Could you check a few things on this model? Use its own coordinates, in mm. A direction names the side the tool comes from. Coordinates: 2 decimals unless noted, no trailing zeros. Write each loop counter-clockwise with the first axis right and the second up, starting at its lowest first coordinate (ties: lowest second). Pieces come first, ordered by that corner, then holes.
Item 1: If I drill on probe 1 along X at (y, z) = (17.5, 9.25); probe 2 along X at (y, z) = (20.5, 3.25), over which ranges is the centre line in solid material (lowest first)?
Item 2: Thinking about a two-plate mould opening in Y: for faces 6 (the cylindrical face through (-22.99, 23.02, 8.3)), 7 (the flat face through (-0.2, 23.2, 10.16)), 8 (the cylindrical face through (-20.609, -17.214, 0.376)), which applies, +Y half, -Y half, draft (parallel to the pull), parting line (faces both ways), or undercut?
Item 3: For P1, Ø5, axis at x = -1.5, y = -7.5, coming from the -Z side; P2, Ø1.2, axis at y = -2, z = 0.5, coming from the -X side; P3, Ø1.7, axis at x = 5.5, z = 0.5, coming from the +Y side; P4, Ø0.8, axis at y = -4.5, z = 2, coming from the -X side, each with a flat end and sliding along its axis, tell me the tip position at first contact or that it passes through.
Item 4: Which directions (+Z, -Z, +X, -X, +Y, -Y) give clear straight access to the entire face, cutting with the end or side of a thin tool? Please do faces 1 (the flat face through (-10, 0, 2.54)), 2 (the flat face through (-6.35, -23, 13)), 3 (the flat face through (0, 22.987, 11)), 4 (the cylindrical face through (-14.86, 13.31, 0.38)), 5 (the flat face through (-25, -19.685, 13)).
Item 5: I want a section at C-C on z = 3.75. Please give me the cut outline in (x, y), then the cut area to 3 significant figures.
Item 6: I want a section at D-D on x = 12. Please give me the cut outline in (y, z) (3 decimals).
Item 7: I want a section at A-A on z = 10.75. State how many separate pieces and enclosed holes the cut face has, then the cut area to 3 significant figures.
from build123d import *

# Parameters (mm, degrees)
BOSS_EXTRUDE1_DEPTH             = 14.224
CUT_EXTRUDE1_DEPTH              = 11.684
FILLET1_R                       = 2.54
CUT_EXTRUDE2_DEPTH              = 55.976332917
CUT_EXTRUDE2_DEPTH_BACK         = 55.976332917
SKETCH3_W                       = 32.258
SKETCH3_H                       = 8.128
SKETCH5_W                       = 26.924
SKETCH5_H                       = 34.29
CUT_EXTRUDE4_DEPTH              = 1.524
SKETCH6_W                       = 16.764
SKETCH6_H                       = 24.13
CUT_EXTRUDE5_DEPTH              = 1.524
SKETCH8_W                       = 12.7
SKETCH8_H                       = 0.508
BOSS_EXTRUDE3_DEPTH             = 4.064
SKETCH9_W                       = 12.7
SKETCH9_H                       = 1.016
BOSS_EXTRUDE4_DEPTH             = 0.762
FILLET2_R                       = 0.762
SKETCH10_W                      = 12.7
SKETCH10_H                      = 1.016
BOSS_EXTRUDE5_DEPTH             = 0.762
FILLET3_R                       = 0.762
SKETCH11_W                      = 1.778
SKETCH11_H                      = 4.064
BOSS_EXTRUDE6_DEPTH             = 3.556
BOSS_EXTRUDE6_DIRECTION_2_REACH = 56.976
FILLET4_RADIUS                  = 2.032
FILLET4_LENGTH                  = 1.778
SKETCH12_R                      = 1.143
CUT_EXTRUDE7_DEPTH              = 4.064
CUT_EXTRUDE8_DEPTH              = 0.762


with BuildPart() as part:
    # Sketch1 → Boss-Extrude1 (new body)
    with BuildSketch(Plane.XY):
        with BuildLine():
            Line((-21.209, -23.749), (21.209, -23.749))
            ThreePointArc((21.209, -23.749), (23.005051224, -23.005051224), (23.749, -21.209))
            Line((23.749, -21.209), (23.749, 21.209))
            ThreePointArc((23.749, 21.209), (23.005051224, 23.005051224), (21.209, 23.749))
            Line((21.209, 23.749), (-21.209, 23.749))
            ThreePointArc((-21.209, 23.749), (-23.005051224, 23.005051224), (-23.749, 21.209))
            Line((-23.749, 21.209), (-23.749, -21.209))
            ThreePointArc((-23.749, -21.209), (-23.005051224, -23.005051224), (-21.209, -23.749))
        make_face()
    extrude(amount=BOSS_EXTRUDE1_DEPTH)

    # Sketch2 → Cut-Extrude1 (cut)
    with BuildSketch(Plane.XY.offset(14.224)):
        with BuildLine():
            Line((19.939, -22.479), (-19.939, -22.479))
            ThreePointArc((-19.939, -22.479), (-21.735051224, -21.735051224), (-22.479, -19.939))
            Line((-22.479, -19.939), (-22.479, 19.939))
            ThreePointArc((-22.479, 19.939), (-21.735051224, 21.735051224), (-19.939, 22.479))
            Line((-19.939, 22.479), (19.939, 22.479))
            ThreePointArc((19.939, 22.479), (21.735051224, 21.735051224), (22.479, 19.939))
            Line((22.479, 19.939), (22.479, -19.939))
            ThreePointArc((22.479, -19.939), (21.735051224, -21.735051224), (19.939, -22.479))
        make_face()
    extrude(amount=-CUT_EXTRUDE1_DEPTH, mode=Mode.SUBTRACT)

    # Fillet1
    fillet1_edges = [part.edges().sort_by_distance(p)[0] for p in [
        (0, -23.749, 0),
        (-23.005051224, -23.005051224, 0),
        (-23.749, 0, 0),
        (-23.005051224, 23.005051224, 0),
        (0, 23.749, 0),
        (23.005051224, 23.005051224, 0),
        (23.749, 0, 0),
        (23.005051224, -23.005051224, 0),
    ]]
    fillet(fillet1_edges, radius=FILLET1_R)

    # Sketch3 → Cut-Extrude2 (cut, two sides: drawn at the far end of the back side and taken through both)
    with BuildSketch(Plane(origin=(0, 23.749, 0), x_dir=(1, 0, 0), z_dir=(0, 1, 0)).offset(-CUT_EXTRUDE2_DEPTH_BACK)):
        with Locations((0, -14.224)):
            Rectangle(SKETCH3_W, SKETCH3_H)
    extrude(amount=CUT_EXTRUDE2_DEPTH + CUT_EXTRUDE2_DEPTH_BACK, mode=Mode.SUBTRACT)

    # Sketch5 → Cut-Extrude4 (cut)
    with BuildSketch(Plane(origin=(0, 0, 0), x_dir=(-1, 0, 0), z_dir=(0, 0, -1))):
        with Locations((-1.143, 0)):
            Rectangle(SKETCH5_W, SKETCH5_H)
    extrude(amount=-CUT_EXTRUDE4_DEPTH, mode=Mode.SUBTRACT)

    # Sketch6 → Cut-Extrude5 (cut)
    with BuildSketch(Plane(origin=(0, 0, 1.524), x_dir=(-1, 0, 0), z_dir=(0, 0, -1))):
        with Locations((-1.143, 0)):
            Rectangle(SKETCH6_W, SKETCH6_H)
    extrude(amount=-CUT_EXTRUDE5_DEPTH, mode=Mode.SUBTRACT)

    # Sketch8 → Boss-Extrude3 (add)
    with BuildSketch(Plane.XY.offset(10.16)):
        with Locations((0, 22.733)):
            Rectangle(SKETCH8_W, SKETCH8_H)
        with Locations((0, -22.733)):
            Rectangle(SKETCH8_W, SKETCH8_H)
    extrude(amount=BOSS_EXTRUDE3_DEPTH)

    # Sketch9 → Boss-Extrude4 (add)
    with BuildSketch(Plane(origin=(0, 22.987, 0), x_dir=(1, 0, 0), z_dir=(0, 1, 0))):
        with Locations((0, -13.716)):
            Rectangle(SKETCH9_W, SKETCH9_H)
    extrude(amount=BOSS_EXTRUDE4_DEPTH)

    # Fillet2
    fillet2_edges = [part.edges().sort_by_distance(p)[0] for p in [
        (0, 22.987, 13.208),
    ]]
    fillet(fillet2_edges, radius=FILLET2_R - 0.0001)  # a hair under: the kernel refuses the full size

    # Sketch10 → Boss-Extrude5 (add)
    with BuildSketch(Plane.XZ.offset(22.987)):
        with Locations((0, 13.716)):
            Rectangle(SKETCH10_W, SKETCH10_H)
    extrude(amount=BOSS_EXTRUDE5_DEPTH)

    # Fillet3
    fillet3_edges = [part.edges().sort_by_distance(p)[0] for p in [
        (0, -22.987, 13.208),
    ]]
    fillet(fillet3_edges, radius=FILLET3_R - 0.0001)  # a hair under: the kernel refuses the full size

    # Sketch11 → Boss-Extrude6 (add)
    with BuildSketch(Plane.ZY.offset(23.749)):
        with Locations((13.335, -21.717)):
            Rectangle(SKETCH11_W, SKETCH11_H)
    extrude(amount=BOSS_EXTRUDE6_DEPTH)

    # Sketch11 → Boss-Extrude6 direction 2 (add, up to next)
    with BuildSketch(Plane.ZY.offset(23.749), mode=Mode.PRIVATE) as boss_extrude6_direction_2_sk1:
        with Locations((13.335, -21.717)):
            Rectangle(SKETCH11_W, SKETCH11_H)
    boss_extrude6_direction_2_tool1 = extrude(boss_extrude6_direction_2_sk1.sketch, amount=-BOSS_EXTRUDE6_DIRECTION_2_REACH, mode=Mode.PRIVATE) - part.part
    add(boss_extrude6_direction_2_tool1.solids().sort_by_distance((-23.749, -21.717, 13.335))[0])

    # Fillet4: full round fillet: the end face becomes a half cylinder, R = half its width
    fillet4_face = Plane((-27.305, -21.717, 13.335), x_dir=(0, 0, -1), z_dir=(-1, 0, 0))  # on the end face: x along it, z out of the body
    fillet4_slab = fillet4_face.offset(-FILLET4_RADIUS / 2) * Box(FILLET4_LENGTH, 2 * FILLET4_RADIUS, FILLET4_RADIUS, mode=Mode.PRIVATE)  # the body's end, R deep
    fillet4_round = Plane((-25.273, -21.717, 13.335), x_dir=(-1, 0, 0), z_dir=(0, 0, -1)) * Cylinder(FILLET4_RADIUS, FILLET4_LENGTH, mode=Mode.PRIVATE)  # its axis R under the face
    add(fillet4_slab - fillet4_round, mode=Mode.SUBTRACT)

    # Sketch12 → Cut-Extrude7 (cut)
    with BuildSketch(Plane(origin=(0, 0, 12.446), x_dir=(-1, 0, 0), z_dir=(0, 0, -1))):
        with Locations((25.273, -21.717)):
            Circle(SKETCH12_R)
    extrude(amount=-CUT_EXTRUDE7_DEPTH, mode=Mode.SUBTRACT)

    # Sketch7 → Cut-Extrude8 (cut)
    with BuildSketch(Plane(origin=(0, 0, 0), x_dir=(-1, 0, 0), z_dir=(0, 0, -1))):
        with BuildLine():
            Line((19.939, 17.145), (21.209, 17.145))
            ThreePointArc((21.209, 17.145), (17.399, 20.955), (13.589, 17.145))
            Line((13.589, 17.145), (14.859, 17.145))
            ThreePointArc((14.859, 17.145), (17.399, 19.685), (19.939, 17.145))
        make_face()
        with BuildLine():
            Line((21.209, 15.875), (16.129, 15.875))
            ThreePointArc((16.129, 15.875), (13.589, 13.335), (16.129, 10.795))
            Line((16.129, 10.795), (21.209, 10.795))
            Line((21.209, 10.795), (21.209, 12.065))
            Line((21.209, 12.065), (16.129, 12.065))
            ThreePointArc((16.129, 12.065), (14.859, 13.335), (16.129, 14.605))
            Line((16.129, 14.605), (21.209, 14.605))
            Line((21.209, 14.605), (21.209, 15.875))
        make_face()
        Polygon((13.589, 9.525), (21.209, 9.525), (21.209, 5.715), (19.939, 5.715), (19.939, 8.255), (18.034, 8.255), (18.034, 6.985), (16.764, 6.985), (16.764, 8.255), (13.589, 8.255), align=None)
        Polygon((13.589, 4.445), (21.209, 4.445), (21.209, 0.635), (19.939, 0.635), (19.939, 3.175), (18.034, 3.175), (18.034, 1.905), (16.764, 1.905), (16.764, 3.175), (13.589, 3.175), align=None)
        Polygon((21.209, -0.635), (13.589, -0.635), (13.589, -4.445), (14.859, -4.445), (14.859, -1.905), (21.209, -1.905), align=None)
        Polygon((13.589, -5.715), (21.209, -5.715), (21.209, -9.525), (19.939, -9.525), (19.939, -6.985), (18.034, -6.985), (18.034, -8.255), (16.764, -8.255), (16.764, -6.985), (14.859, -6.985), (14.859, -9.525), (13.589, -9.525), align=None)
        with BuildLine():
            Line((18.9865, -13.97), (18.9865, -15.24))
            ThreePointArc((18.9865, -15.24), (20.558044821, -11.445955179), (16.764, -13.0175))
            ThreePointArc((16.764, -13.0175), (15.137980791, -13.691019209), (15.8115, -12.065))
            Line((15.8115, -12.065), (15.8115, -10.795))
            ThreePointArc((15.8115, -10.795), (14.239955179, -14.589044821), (18.034, -13.0175))
            ThreePointArc((18.034, -13.0175), (19.660019209, -12.343980791), (18.9865, -13.97))
        make_face()
        with BuildLine():
            Line((15.8115, -17.78), (15.8115, -16.51))
            ThreePointArc((15.8115, -16.51), (14.239955179, -20.304044821), (18.034, -18.7325))
            ThreePointArc((18.034, -18.7325), (19.660019209, -18.058980791), (18.9865, -19.685))
            Line((18.9865, -19.685), (18.9865, -20.955))
            ThreePointArc((18.9865, -20.955), (20.558044821, -17.160955179), (16.764, -18.7325))
            ThreePointArc((16.764, -18.7325), (15.137980791, -19.406019209), (15.8115, -17.78))
        make_face()
    extrude(amount=-CUT_EXTRUDE8_DEPTH, mode=Mode.SUBTRACT)


solid = part.part
Response values:
1. probe 1: x = -23.75 to -22.48, 22.48 to 23.75
1. probe 2: x = -23.75 to -22.42, 22.42 to 23.75
2. face 6: +Y half
2. face 7: draft
2. face 8: undercut
3. P1: passes through
3. P2: stops at x = -23.3
3. P3: stops at y = 23.45
3. P4: stops at x = -23.75
4. face 1: +Z
4. face 2: +Z, +Y, -Y
4. face 3: +Y
4. face 4: -Z
4. face 5: +Z, -Z, -X, +Y
5. outline: (-23.75, -21.21) arc R2.54 ccw to (-21.21, -23.75) - (21.21, -23.75) arc R2.54 ccw to (23.75, -21.21) - (23.75, 21.21) arc R2.54 ccw to (21.21, 23.75) - (-21.21, 23.75) arc R2.54 ccw to (-23.75, 21.21) - close; hole (-22.48, -19.94) arc R2.54 ccw to (-19.94, -22.48) - (19.94, -22.48) arc R2.54 ccw to (22.48, -19.94) - (22.48, 19.94) arc R2.54 ccw to (19.94, 22.48) - (-19.94, 22.48) arc R2.54 ccw to (-22.48, 19.94) - close
5. area: 235 mm2
6. outline: (-23.749, 2.54) arc R2.54 ccw to (-21.209, 0) - (-17.145, 0) - (-17.145, 1.524) - (17.145, 1.524) - (17.145, 0) - (21.209, 0) arc R2.54 ccw to (23.749, 2.54) - (23.749, 10.16) - (22.479, 10.16) - (22.479, 2.54) - (-22.479, 2.54) - (-22.479, 10.16) - (-23.749, 10.16) - close
7. separate pieces: 4
7. enclosed holes: 0
7. area: 166 mm2
